Can you work these out from the model? Positions are in its coordinate system, mm. Face numbers are marked on the shaded views. A direction names the side the tool comes from. Give positions to 0.01 mm unless a question says otherwise; leave off trailing zeros. Loops run counter-clockwise (first coordinate to the right, second up) from the corner with the lowest first, then second, coordinate; pieces in that order, holes last. Notation, with made-up numbers: M -26,49 L -3,49 A17 cw -3,64 Z; hole C 34,40 d3. An arc over 180 degrees is marked long. Answer as a JSON object with one key per item and string values.
```python
from build123d import *


with BuildPart() as part:
    # Çizim2 → Döndür2 (revolve)
    with BuildSketch(Plane(origin=(0, 0, 0), x_dir=(0, 0, -1), z_dir=(0, 1, 0)), mode=Mode.PRIVATE) as d_nd_r2_sk:
        with BuildLine():
            Line((-2.5, 2.9), (2.5, 2.9))
            Line((2.5, 2.9), (2.5, 4.9))
            ThreePointArc((2.5, 4.9), (2.207106781, 5.607106781), (1.5, 5.9))
            Line((1.5, 5.9), (1, 5.9))
            Line((1, 5.9), (1, 3.9))
            Line((1, 3.9), (-1, 3.9))
            Line((-1, 3.9), (-1, 5.9))
            Line((-1, 5.9), (-1.5, 5.9))
            ThreePointArc((-1.5, 5.9), (-2.207106781, 5.607106781), (-2.5, 4.9))
            Line((-2.5, 4.9), (-2.5, 2.9))
        make_face()
    revolve(d_nd_r2_sk.sketch.rotate(Axis((0, 0, 0), (0, 0, -1)), 180), axis=Axis((0, 0, 0), (0, 0, -1)))


solid = part.part
```
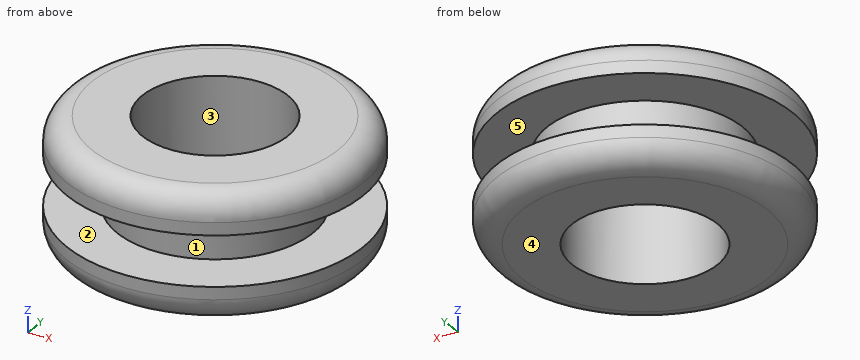
1) Will these pins go through, and if not, where does the flat tip stop? pin 1 Ø3 at (x, z) = (0.5, 1) entering from +Y; pin 2 Ø1.5 at (x, z) = (2, -0.5) entering from -Y.
Answer list:
{"pin 1": "y = 5.9", "pin 2": "y = -5.72"}
2) If we mould it in two halves opening along Y, with no side actions, what happens to the marked faces 1, 2 and 3? For each: +Y half, -Y half, draft (parallel to the pull), parting line (faces both ways), or undercut.
Answer list:
{"face 1": "parting line", "face 2": "draft", "face 3": "undercut"}
3) Suppose I cut it at D-D, the plane z = 1.8. Write out the boundary of the cut face in (x, y), and give its area (3 significant figures).
Answer list:
{"outline": "C 0,0 d11.71; hole C 0,0 d5.8", "area": "81.2 mm^2"}
4) Suppose I cut it at A-A, the plane x = 0. Write out the boundary of the cut face in (y, z).
Answer list:
{"outline": "M -5.9,-1.5 A1 ccw -4.9,-2.5 L -2.9,-2.5 L -2.9,2.5 L -4.9,2.5 A1 ccw -5.9,1.5 L -5.9,1 L -3.9,1 L -3.9,-1 L -5.9,-1 Z; M 2.9,-2.5 L 4.9,-2.5 A1 ccw 5.9,-1.5 L 5.9,-1 L 3.9,-1 L 3.9,1 L 5.9,1 L 5.9,1.5 A1 ccw 4.9,2.5 L 2.9,2.5 Z"}
5) For the marked faces 4 and 5, which set-ups out of +Z, -Z, +X, -X, +Y, -Y let a thin tool reach every point of the face, with its end or its side?
Answer list:
{"face 4": "-Z, +X, -X, +Y, -Y", "face 5": "none"}
6) Suppose I cut it at C-C, the plane z = 0.8. Write out the boundary of the cut face in (x, y).
Answer list:
{"outline": "C 0,0 d7.8; hole C 0,0 d5.8"}
7) Please list where these lines run through material, in increasing order: line 1 along Y through (x, z) = (0, -0.25); line 2 along Z through (x, y) = (-3, 3.75); line 3 along Y through (x, z) = (0, -1.5). Write a range as from..to.
Answer list:
{"line 1": "-3.9..-2.9, 2.9..3.9", "line 2": "-2.5..-1, 1..2.5", "line 3": "-5.9..-2.9, 2.9..5.9"}
